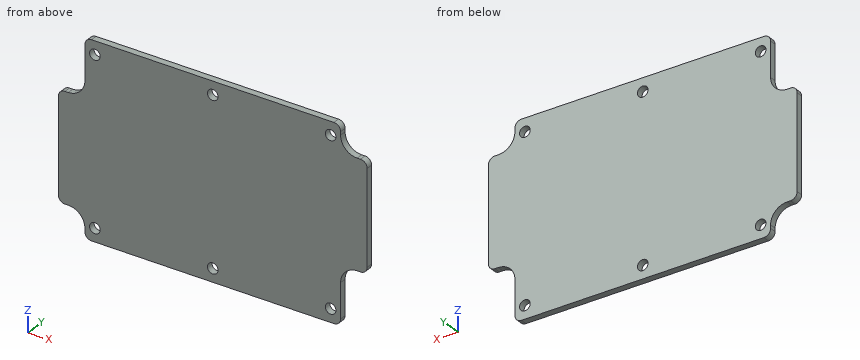
Autodesk Inventor part; units mm, degrees
ref_plane "XZ Plane" through (0, 0, 0) normal (0, 1, 0) x (-1, 0, 0)
sketch "Sketch1" plane through (0, 0, 0) normal (0, 1, 0) x (-1, 0, 0)
  line L0 (-36.5, 29) -> (36.5, 29)
  line L1 (38.5, 27) -> (38.5, 16.5)
  line L2 (43.5, 11.5) -> (44.5, 11.5)
  line L3 (46.5, 9.5) -> (46.5, -19)
  line L4 (44.5, -21) -> (43.5, -21)
  line L5 (38.5, -26) -> (38.5, -27)
  line L6 (36.5, -29) -> (-36.5, -29)
  line L7 (0, 29) -> (0, -29) construction
  arc A0 (44.5, -21) -> (46.5, -19) centre (44.5, -19) ccw
  arc A1 (36.5, -29) -> (38.5, -27) centre (36.5, -27) ccw
  arc A2 (43.5, -21) -> (38.5, -26) centre (43.5, -26) ccw
  arc A3 (38.5, 16.5) -> (43.5, 11.5) centre (43.5, 16.5) ccw
  arc A4 (38.5, 27) -> (36.5, 29) centre (36.5, 27) ccw
  arc A5 (46.5, 9.5) -> (44.5, 11.5) centre (44.5, 9.5) ccw
  line L8 (-38.5, 27) -> (-38.5, 26)
  line L9 (-43.5, 21) -> (-44.5, 21)
  line L10 (-46.5, 19) -> (-46.5, -9.5)
  line L11 (-44.5, -11.5) -> (-43.5, -11.5)
  line L12 (-38.5, -16.5) -> (-38.5, -27)
  arc A6 (-36.5, 29) -> (-38.5, 27) centre (-36.5, 27) ccw
  arc A7 (-44.5, 21) -> (-46.5, 19) centre (-44.5, 19) ccw
  arc A8 (-46.5, -9.5) -> (-44.5, -11.5) centre (-44.5, -9.5) ccw
  arc A9 (-38.5, -27) -> (-36.5, -29) centre (-36.5, -27) ccw
  arc A10 (-43.5, 21) -> (-38.5, 26) centre (-43.5, 26) ccw
  arc A11 (-38.5, -16.5) -> (-43.5, -11.5) centre (-43.5, -16.5) ccw
  point P0 (0, 0)
  point P1 (38.5, 29)
  point P2 (38.5, -21)
  point P3 (38.5, -29)
  point P4 (0, 0)
  point P5 (-38.5, -11.5)
  dimension "d0" = 8
  dimension "d2" = 8
  dimension "d3" = 2
  dimension "d4" = 5
  dimension "d5" = 17.5
  dimension "d6" = 5
  dimension "d7" = 2
  dimension "d8" = 58
  dimension "d9" = 8
  dimension "d10" = 17.5
  dimension "d11" = 8
  dimension "d12" = 93
  dimension "d13" = 2
  dimension "d14" = 5
extrude "Extrusion1" add sketch "Sketch1" along normal blind 2
sketch "Sketch2" plane through (0, 2, 0) normal (0, 1, 0) x (1, 0, 0)
  line L0 (35.5, 25) -> (-35.5, 25) construction
  line L1 (-35.5, 25) -> (-35.5, -25) construction
  line L2 (-35.5, -25) -> (35.5, -25) construction
  line L3 (35.5, -25) -> (35.5, 25) construction
  line L4 (35.5, 25) -> (-35.5, -25) construction
  line L5 (-35.5, 25) -> (35.5, -25) construction
  point P0 (0, 0)
  point P1 (0, -25)
  point P2 (0, 25)
  point P3 (0, 25)
  point P4 (0, -25)
  dimension "d17" = 35.5
  dimension "d18" = 50
hole "Hole1" at (0, 2, 25) at (-35.5, 2, 25) at (-35.5, 2, -25) at (0, 2, -25) at (35.5, 2, 25) at (35.5, 2, -25) direction (0, -1, 0) diameter 3.2 depth 7.5
equation "\"d2\" = d0"
equation "\"d6\" = d4"
equation "\"d7\" = d3"
equation "\"d9\" = d0"
equation "\"d10\" = d5"
equation "\"d11\" = d0"
equation "\"d13\" = d3"
equation "\"d14\" = d4"
properties part number "CH_01_0042_pcb_layout"
The model under review builds one solid part; all positions refer to its coordinate system, in mm. Give positions to 0.01 mm unless a question says otherwise; leave off trailing zeros. Loops run counter-clockwise (first coordinate to the right, second up) from the corner with the lowest first, then second, coordinate; pieces in that order, holes last. Notation, with made-up numbers: (3, 43) -> (20, 43) arc R24 ccw to (20, 62) -> close; hole circle Ø8 at (58.5, -10.75). An arc over 180 degrees is marked (long way). Answer as a JSON object with one key per item and string values. Group by question number.
Q1. Take a section at B-B (x = 0). Write out the cut boundary in (y, z).
Q2. Wall thickness on line 1 along Z through (x, y) = (0, 0.6); line 2 along X through (y, z) = (0.65, 25); line 3 along X through (y, z) = (0.6, -25): over which ranges is each line inside the solid? List them lowest first.
Q3. Take a section at A-A (y = 0.9). State how many separate pieces and enclosed holes the cut face has, plus the area to 3 significant figures.
Q4. Insertion check: pin 1 (1 mm diameter, centred on x = 18.5, z = -19.5, fed in from -Y); pin 2 (0.5 mm diameter, centred on y = 1.5, z = -26.5, fed in from -X); pin 3 (1 mm diameter, centred on y = 1, z = -20, fed in from +X); pin 4 (0.8 mm diameter, centred on x = 44, y = 1, fed in from -Z). Each pin has a flat end and moves straight along its axis. Give the tip position at first contact, or say it passes through.
Q5. Take a section at C-C (z = 25). Write out the cut boundary in (x, y), plus the area to 3 significant figures.
Q6. Take a section at D-D (z = -22). Write out the cut boundary in (x, y).
Answer below:
{
 "1": {"outline": "(0, -29) -> (2, -29) -> (2, -26.6) -> (0, -26.6) -> close; (0, -23.4) -> (2, -23.4) -> (2, 23.4) -> (0, 23.4) -> close; (0, 26.6) -> (2, 26.6) -> (2, 29) -> (0, 29) -> close"},
 "2": {"line 1": "z = -29 to -26.6, -23.4 to 23.4, 26.6 to 29", "line 2": "x = -38.5 to -37.1, -33.9 to -1.6, 1.6 to 33.9, 37.1 to 38.6", "line 3": "x = -38.6 to -37.1, -33.9 to -1.6, 1.6 to 33.9, 37.1 to 38.5"},
 "3": {"separate pieces": "1", "enclosed holes": "6", "area": "4,950 mm2"},
 "4": {"pin 1": "stops at y = 0", "pin 2": "stops at x = -38.5", "pin 3": "stops at x = 38.5", "pin 4": "stops at z = -11.5"},
 "5": {"outline": "(-38.5, 0) -> (-37.1, 0) -> (-37.1, 2) -> (-38.5, 2) -> close; (-33.9, 0) -> (-1.6, 0) -> (-1.6, 2) -> (-33.9, 2) -> close; (1.6, 0) -> (33.9, 0) -> (33.9, 2) -> (1.6, 2) -> close; (37.1, 0) -> (38.6, 0) -> (38.6, 2) -> (37.1, 2) -> close", "area": "135 mm2"},
 "6": {"outline": "(-40.5, 0) -> (38.5, 0) -> (38.5, 2) -> (-40.5, 2) -> close"}
}
